Could you check a few things on this model? Use its own coordinates, in mm. A direction names the side the tool comes from. Round coordinates to 2 decimals unless told otherwise and drop trailing zeros. Order: outer loops, then holes, each group sorted by start corner. A loop starts at its lowest first (then second) coordinate and runs counter-clockwise, first axis right, second up. Notation, with made-up numbers: (34, 48) - (63, 48) arc R17 cw to (63, 53) - close; hole circle Ø8 at (5.25, 60). An arc over 180 degrees is marked (long way). Return JSON: item names as keys, results as strings. Group by question number.
from build123d import *

# Parameters (mm, degrees)
SKETCH2_W       = 3
SKETCH2_H       = 0.7
SLOT_DEPTH      = 0.5
THDSCHPAT_COUNT = 16
THDSCHPAT_PITCH = 0.4


with BuildPart() as part:
    # BodySke → Base-Revolve (revolve)
    with BuildSketch(Plane.XY, mode=Mode.PRIVATE) as base_revolve_sk:
        with BuildLine():
            Line((1.6, 0.9), (1.6, 1.5))
            Line((1.6, 1.5), (0.8, 1.5))
            ThreePointArc((0.8, 1.5), (0.234314575, 1.265685425), (0, 0.7))
            Line((0, 0.7), (0, 0))
            Line((0, 0), (9.1, 0))
            Line((9.1, 0), (9.1, 0.9))
            Line((9.1, 0.9), (1.6, 0.9))
        make_face()
    revolve(base_revolve_sk.sketch.rotate(Axis((-25.4, 0, 0), (1, 0, 0)), 90), axis=Axis((-25.4, 0, 0), (1, 0, 0)))

    # Sketch2 → Slot (cut)
    with BuildSketch(Plane(origin=(0, 0, 0), x_dir=(0, 0, -1), z_dir=(1, 0, 0))):
        Rectangle(SKETCH2_W, SKETCH2_H)
    extrude(amount=SLOT_DEPTH, mode=Mode.SUBTRACT)

    # ThdSchSke → ThreadSchematic (revolve, cut)
    with BuildSketch(Plane.XY, mode=Mode.PRIVATE) as threadschematic_sk:
        Polygon((3.1, -0.774), (3.01177385, -0.9), (3.01177385, -1.35), (3.18822615, -1.35), (3.18822615, -0.9), align=None)
    threadschematic = revolve(threadschematic_sk.sketch.rotate(Axis((-3.175, 0, 0), (1, 0, 0)), 270), axis=Axis((-3.175, 0, 0), (1, 0, 0)), mode=Mode.SUBTRACT)

    # ThdSchPat: ThreadSchematic ×16
    with Locations(*[(i * THDSCHPAT_PITCH, 0, 0) for i in range(1, THDSCHPAT_COUNT)]):
        add(threadschematic, mode=Mode.SUBTRACT)


solid = part.part
1) For faces 1 (the cylindrical face through (2.3, -0.27, 0.86)), 2 (the cylindrical face through (1.19, -0.45, 1.43)), which set-ups out of +Z, -Z, +X, -X, +Y, -Y let a thin tool reach every point of the face, with its end or its side?
2) I want a section at A-A, the plane x = 1. List the corners of the cut face in (y, z) for me, plus the area to 3 significant figures.
3) Will these pins go through, and if not, where does the flat tip stop? pin 1 (0.6 mm diameter, centred on x = 0, z = 0.5, fed in from +Y); pin 2 (1.5 mm diameter, centred on x = 3, z = -1, fed in from -Y).
4) If I drill on line 1 along X through (y, z) = (0, 0.2); line 2 along X through (y, z) = (-0.75, -0.55); line 3 along Y through (x, z) = (1.5, -0.6), over which ranges is the centre line in solid material (lowest first)? Write a range as from..to.
Outcome:
{
 "1": {"face 1": "+X", "face 2": "+X, -X"},
 "2": {"outline": "circle Ø3 at (0, 0)", "area": "7.07 mm^2"},
 "3": {"pin 1": "y = 1.25", "pin 2": "y = -0.86"},
 "4": {"line 1": "0.5..9.1", "line 2": "0.03..1.6", "line 3": "-1.37..1.37"}
}
